from build123d import *

# Parameters (mm, degrees)
F0_W          = 100
F0_H          = 100
F0_W_2        = 82
F0_H_2        = 25
F1_DEPTH      = 16.5
F2_DEPTH      = 34
F4_DEPTH      = 100.001
F6_DEPTH      = 50.001
F6_DEPTH_BACK = 50.001
F7_W          = 70
F7_H          = 16
F8_DEPTH      = 16.501


with BuildPart() as f1:
    # F0 (on Top) → F1 (new body)
    with BuildSketch(Plane.XY):
        Rectangle(F0_W, F0_H)
        Rectangle(F0_W_2, F0_H_2, mode=Mode.SUBTRACT)
        Rectangle(F0_W_2, F0_H_2)
    extrude(amount=-F1_DEPTH)

    # F0 (on Top) → F2 (join)
    with BuildSketch(Plane.XY):
        Rectangle(F0_W, F0_H)
        Rectangle(F0_W_2, F0_H_2, mode=Mode.SUBTRACT)
    extrude(amount=F2_DEPTH)

    # F3 (on face) → F4 (cut, through all)
    with BuildSketch(Plane(origin=(-50, 0, 0), x_dir=(0, -1, 0), z_dir=(-1, 0, 0))):
        Polygon((50, 34), (14.5, 34), (22.1871227195, -9.5958393243), (50, -14.5), align=None)
        Polygon((-22.1871227195, -9.5958393243), (-14.5, 34), (-50, 34), (-50, -14.5), align=None)
    extrude(amount=-F4_DEPTH, mode=Mode.SUBTRACT)

    # F5 (on Front) → F6 (cut, two sides)
    with BuildSketch(Plane.XZ) as f6_sk:
        Polygon((-50, -14.5), (-43, 34), (-50, 34), align=None)
        Polygon((50, 34), (43, 34), (50, -14.5), align=None)
    extrude(amount=-F6_DEPTH, mode=Mode.SUBTRACT)
    extrude(f6_sk.sketch, amount=F6_DEPTH_BACK, mode=Mode.SUBTRACT)

    # F7 (on face) → F8 (cut, through all)
    with BuildSketch(Plane.XY):
        Rectangle(F7_W, F7_H)
    extrude(amount=-F8_DEPTH, mode=Mode.SUBTRACT)


solid = f1.part
Input: part model. Units: mm. Frame: model coordinates. A direction names the side the tool comes from. Give positions to 0.01 mm unless a question says otherwise; leave off trailing zeros. Write each loop counter-clockwise with the first axis right and the second up, starting at its lowest first coordinate (ties: lowest second). Pieces come first, ordered by that corner, then holes. Notation, with made-up numbers: M 68,-8.5 L 73,-8.5 A21 ccw 73,23.5 Z; hole C -26,15 d6. An arc over 180 degrees is marked long. Write item = value, one per line. Start each with the question number.
1) Cut plane A-A on y = -6. Return the cut outline in (x, z).
2) Cut plane B-B on x = -28.5. Return the cut outline in (y, z), then the cut area to 3 significant figures.
3) First-contact query: pin 1 Ø7.5 at (y, z) = (-0.5, 11.5) entering from +X; pin 2 Ø4 at (x, z) = (-24.5, 20.5) entering from -Y; pin 3 Ø5 at (y, z) = (4, -7.5) entering from +X. Flat tips, straight axial feed; report the tip coordinate or a pass-through.
4) Reachability of faces 1 (the flat face through (41, 0, 17)), 2 (the flat face through (0, -8, -8)), 3 (the flat face through (-0.7, -35.899, -12.014)) from +Z, -Z, +X, -X, +Y, -Y: full face, straight path, thin tool, end or side. Return the list, or none.
5) Cut plane C-C on z = -5.5. Return the cut outline in (x, y), then the cut area to 3 significant figures.
6) Draft query along Y for faces 4 (the flat face through (-0.69, -18.29, 12.51)), 5 (the flat face through (-0.69, 18.397, 11.897)), 6 (the flat face through (0, 8, -8)). Return one class per face: +Y half, -Y half, draft (parallel to the pull), parting line (faces both ways), or undercut.
7) Material intervals for line 1 along Y through (x, z) = (-32, 9); line 2 along Y through (x, z) = (-10, 15.5); line 3 along X through (y, z) = (-6, -5.5), sorted ascending. Write a range as [from, to].
8) Cut plane D-D on y = 10.5. Return the cut outline in (x, z).
Solved:
q1.outline = M -50,-16.5 L -35,-16.5 L -35,0 L -41,0 L -41,34 L -43,34 L -50,-14.5 Z; M 35,-16.5 L 50,-16.5 L 50,-14.5 L 43,34 L 41,34 L 41,0 L 35,0 Z
q2.outline = M -50,-16.5 L -8,-16.5 L -8,0 L -12.5,0 L -12.5,34 L -14.5,34 L -22.19,-9.6 L -50,-14.5 Z; M 8,-16.5 L 50,-16.5 L 50,-14.5 L 22.19,-9.6 L 14.5,34 L 12.5,34 L 12.5,0 L 8,0 Z
q2.area = 1,040 mm2
q3.pin_1 = 46.79
q3.pin_2 = -17.23
q3.pin_3 = 49.35
q4.face_1 = +Z
q4.face_2 = +Z, -Z
q4.face_3 = +Z, +X, -X, -Y
q5.outline = M -48.7,-21.46 L 48.7,-21.46 L 48.7,21.46 L -48.7,21.46 Z; hole M -35,-8 L 35,-8 L 35,8 L -35,8 Z
q5.area = 3,060 mm2
q6.face_4 = -Y half
q6.face_5 = +Y half
q6.face_6 = undercut
q7.line_1 = [-18.91, -12.5], [12.5, 18.91]
q7.line_2 = [-17.76, -12.5], [12.5, 17.76]
q7.line_3 = [-48.7, -35], [35, 48.7]
q8.outline = M -50,-16.5 L 50,-16.5 L 50,-14.5 L 43,34 L 41,34 L 41,0 L -41,0 L -41,34 L -43,34 L -50,-14.5 Z
